```python
from build123d import *

# Parameters (mm, degrees)
SKETCH_1_W          = 196
SKETCH_1_H          = 221
EXTRUDE_1_DEPTH     = 3
EXTRUDE_2_DEPTH     = 128
FILLET_1_R          = 10
FILLET_2_R          = 10
SKETCH_3_R          = 3
SKETCH_3_R_2        = 40
CUT_EXTRUDE_1_DEPTH = 5
FILLET_3_R          = 10
FILLET_4_R          = 10
SKETCH_5_R          = 40
SKETCH_5_R_2        = 34
EXTRUDE_3_DEPTH     = 3
SKETCH_6_W          = 15
SKETCH_6_H          = 9
CUT_EXTRUDE_3_DEPTH = 159
EXTRUDE_4_DEPTH     = 10
EXTRUDE_4_2_DEPTH   = 10
EXTRUDE_4_3_DEPTH   = 10
EXTRUDE_4_4_DEPTH   = 10
EXTRUDE_6_DEPTH     = 1.5
FILLET_START        = -219
FILLET_6_DEPTH      = 216
FILLET_7_R          = 6.5
FILLET_8_R          = 8.5
FILLET_9_R          = 8.5
CUT_EXTRUDE_4_DEPTH = 10


with BuildPart() as part:
    # Sketch 1 → Extrude 1 (new body)
    with BuildSketch(Plane(origin=(0, 0, 0), x_dir=(1, 0, 0), z_dir=(0, 1, 0))):
        with Locations((98, 110.5)):
            Rectangle(SKETCH_1_W, SKETCH_1_H)
    extrude(amount=EXTRUDE_1_DEPTH)

    # Sketch 2 → Extrude 2 (add)
    with BuildSketch(Plane(origin=(0, 0, 0), x_dir=(1, 0, 0), z_dir=(0, 1, 0))):
        Polygon((3, 218), (3, 3), (20.5, 3), (20.5, 18), (24.5, 18), (24.5, 3), (24.5, 0), (0, 0), (0, 221), (196, 221), (196, 0), (171.5, 0), (171.5, 3), (171.5, 18), (175.5, 18), (175.5, 3), (193, 3), (193, 218), align=None)
    extrude(amount=-EXTRUDE_2_DEPTH)

    # Fillet 1
    fillet_1_edges = [part.edges().sort_by_distance(p)[0] for p in [
        (0, 3, -110.5),
    ]]
    fillet(fillet_1_edges, radius=FILLET_1_R)

    # Fillet 2
    fillet_2_edges = [part.edges().sort_by_distance(p)[0] for p in [
        (196, 3, -110.5),
    ]]
    fillet(fillet_2_edges, radius=FILLET_2_R)

    # Sketch 3 → Cut-Extrude 1 (cut)
    with BuildSketch(Plane(origin=(0, 0, -221), x_dir=(-1, 0, 0), z_dir=(0, 0, -1))):
        with Locations((-133.75, -9)):
            Circle(SKETCH_3_R)
        with Locations((-62.25, -9)):
            Circle(SKETCH_3_R)
        with Locations((-62.25, -80.5)):
            Circle(SKETCH_3_R)
        with Locations((-133.75, -80.5)):
            Circle(SKETCH_3_R)
        with Locations((-98, -44.75)):
            Circle(SKETCH_3_R_2)
    extrude(amount=-CUT_EXTRUDE_1_DEPTH, mode=Mode.SUBTRACT)

    # Fillet 3
    fillet_3_edges = [part.edges().sort_by_distance(p)[0] for p in [
        (193, 0, -110.5),
    ]]
    fillet(fillet_3_edges, radius=FILLET_3_R)

    # Fillet 4
    fillet_4_edges = [part.edges().sort_by_distance(p)[0] for p in [
        (3, 0, -110.5),
    ]]
    fillet(fillet_4_edges, radius=FILLET_4_R)

    # Sketch 5 → Extrude 3 (add)
    with BuildSketch(Plane(origin=(0, 0, -221), x_dir=(-1, 0, 0), z_dir=(0, 0, -1))):
        with Locations((-98, -44.75)):
            Circle(SKETCH_5_R)
        with Locations((-98, -44.75)):
            Circle(SKETCH_5_R_2, mode=Mode.SUBTRACT)
    extrude(amount=-EXTRUDE_3_DEPTH)

    # Sketch 6 → Cut-Extrude 3 (cut)
    with BuildSketch(Plane(origin=(175.5, 0, 0), x_dir=(0, 0, -1), z_dir=(1, 0, 0))):
        with Locations((10.5, -123.5)):
            Rectangle(SKETCH_6_W, SKETCH_6_H)
    extrude(amount=-CUT_EXTRUDE_3_DEPTH, mode=Mode.SUBTRACT)



with BuildPart() as body_2:
    # Sketch 10 → Extrude 4 (new body)
    with BuildSketch(Plane(origin=(0, -128, 0), x_dir=(-1, 0, 0), z_dir=(0, -1, 0))):
        Polygon((-5.5, 213.5), (-5.5, 143.5), (-9.5, 143.5), (-9.5, 209.5), (-35.5, 209.5), (-35.5, 213.5), align=None)
    extrude(amount=-EXTRUDE_4_DEPTH)


with BuildPart() as body_3:
    # Sketch 10 → Extrude 4 2 (new body)
    with BuildSketch(Plane(origin=(0, -128, 0), x_dir=(-1, 0, 0), z_dir=(0, -1, 0))):
        Polygon((-190.5, 213.5), (-160.5, 213.5), (-160.5, 209.5), (-186.5, 209.5), (-186.5, 143.5), (-190.5, 143.5), align=None)
    extrude(amount=-EXTRUDE_4_2_DEPTH)


with BuildPart() as body_4:
    # Sketch 10 → Extrude 4 3 (new body)
    with BuildSketch(Plane(origin=(0, -128, 0), x_dir=(-1, 0, 0), z_dir=(0, -1, 0))):
        Polygon((-16.5, 6.5), (-16.5, 10.5), (-9.5, 10.5), (-9.5, 116.5), (-5.5, 116.5), (-5.5, 6.5), align=None)
    extrude(amount=-EXTRUDE_4_3_DEPTH)


with BuildPart() as body_5:
    # Sketch 10 → Extrude 4 4 (new body)
    with BuildSketch(Plane(origin=(0, -128, 0), x_dir=(-1, 0, 0), z_dir=(0, -1, 0))):
        Polygon((-190.5, 6.5), (-179.5, 6.5), (-179.5, 10.5), (-186.5, 10.5), (-186.5, 116.5), (-190.5, 116.5), align=None)
    extrude(amount=-EXTRUDE_4_4_DEPTH)


with BuildPart() as part_1:
    add(part.part)

    add(body_2.part)  # Extrude 6 merges body 2

    add(body_3.part)  # Extrude 6 merges body 3

    add(body_4.part)  # Extrude 6 merges body 4

    add(body_5.part)  # Extrude 6 merges body 5
    # Sketch 11 → Extrude 6 (add)
    with BuildSketch(Plane(origin=(0, -118, 0), x_dir=(1, 0, 0), z_dir=(0, 1, 0))):
        Polygon((179.5, 6.5), (179.5, 3), (193, 3), (193, 218), (160.5, 218), (160.5, 209.5), (186.5, 209.5), (186.5, 10.5), (179.5, 10.5), align=None)
        Polygon((16.5, 10.5), (16.5, 3), (3, 3), (3, 218), (35.5, 218), (35.5, 209.5), (9.5, 209.5), (9.5, 10.5), align=None)
    extrude(amount=EXTRUDE_6_DEPTH)

    # Fillet 6: read off the stored shape, not the designer's step
    # Fillet 6 outline → Fillet 6 (add)
    with BuildSketch(Plane.XY.offset(FILLET_START)):
        with BuildLine():
            Line((3, -116.5), (9.5, -116.5))
            ThreePointArc((9.5, -116.5), (4.903805922, -114.596194078), (3, -110))
            Line((3, -110), (3, -116.5))
        make_face()
    extrude(amount=FILLET_6_DEPTH)

    # Fillet 7
    fillet_7_edges = [part_1.edges().sort_by_distance(p)[0] for p in [
        (193, -116.5, -110.5),
    ]]
    fillet(fillet_7_edges, radius=FILLET_7_R - 0.0001)  # a hair under: the kernel refuses the full size

    # Fillet 8
    # the kernel refuses this fillet: 8.5 mm, written as the material it adds along each edge
    with BuildSketch(Plane(origin=(-11.75, -116.5, -218), x_dir=(0, 1, 0), z_dir=(1, 0, 0))) as fillet_8_piece_1_section:
        with BuildLine():
            CenterArc((FILLET_8_R, FILLET_8_R), FILLET_8_R, 180, 90)
            Line((0, FILLET_8_R), (0, 0))
            Line((0, 0), (FILLET_8_R, 0))
        make_face()
    fillet_8_piece_1 = extrude(amount=47.25, mode=Mode.PRIVATE)
    fillet_8_piece_1 = split(fillet_8_piece_1, bisect_by=Plane(origin=(0, -116.5, -218), z_dir=(1, 0, 0)), keep=Keep.TOP, mode=Mode.PRIVATE)
    add(fillet_8_piece_1)

    # Fillet 9
    # the kernel refuses this fillet: 8.5 mm, written as the material it adds along each edge
    with BuildSketch(Plane(origin=(207.7501, -116.5, -218), x_dir=(0, 0, 1), z_dir=(-1, 0, 0))) as fillet_9_piece_1_section:
        with BuildLine():
            CenterArc((FILLET_9_R, FILLET_9_R), FILLET_9_R, 180, 90)
            Line((0, FILLET_9_R), (0, 0))
            Line((0, 0), (FILLET_9_R, 0))
        make_face()
    fillet_9_piece_1 = extrude(amount=47.2501, mode=Mode.PRIVATE)
    fillet_9_piece_1 = split(fillet_9_piece_1, bisect_by=Plane(origin=(196, -116.5, -218), z_dir=(-1, 0, 0)), keep=Keep.TOP, mode=Mode.PRIVATE)
    add(fillet_9_piece_1)

    # Sketch 12 → Cut-Extrude 4 (cut)
    with BuildSketch(Plane(origin=(0, -128, 0), x_dir=(-1, 0, 0), z_dir=(0, -1, 0))):
        Polygon((-16.5, 6.5), (-5.5, 6.5), (-5.5, 213.5), (-35.5, 213.5), (-35.5, 212.5), (-6.5, 212.5), (-6.5, 7.5), (-16.5, 7.5), align=None)
        Polygon((-190.5, 213.5), (-190.5, 6.5), (-179.5, 6.5), (-179.5, 7.5), (-189.5, 7.5), (-189.5, 212.5), (-160.5, 212.5), (-160.5, 213), (-160.5, 213.5), align=None)
    extrude(amount=-CUT_EXTRUDE_4_DEPTH, mode=Mode.SUBTRACT)


solid = part_1.part
```
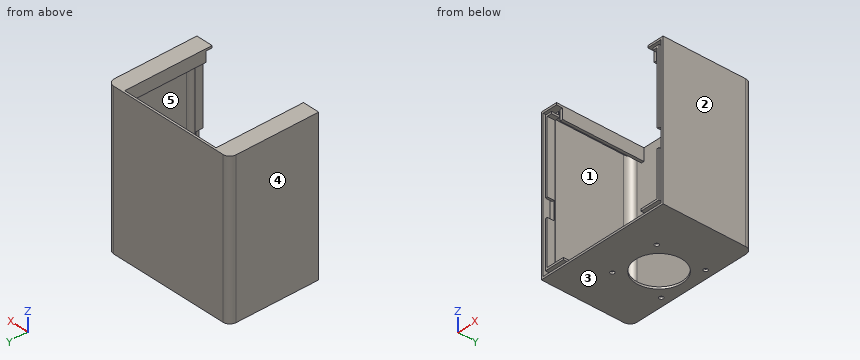
Design review of the part built by this model. Coordinates are the model's own, in mm. Face numbers are marked on the shaded views. A direction names the side the tool comes from. Give positions to 0.01 mm unless a question says otherwise; leave off trailing zeros. Write each loop counter-clockwise with the first axis right and the second up, starting at its lowest first coordinate (ties: lowest second). Pieces come first, ordered by that corner, then holes.
(1) Add section D-D (x = 74). Give the boundary of the cut face in (y, z).
Checked values:
outline: (-128, -221) - (-68.83, -221) - (-68.83, -218) - (-128, -218) - close; (-20.67, -221) - (3, -221) - (3, 0) - (0, 0) - (0, -218) - (-20.67, -218) - close
(2) Mouldability with a two-part tool opening along Z and no side actions: class the marked faces 3, 4 and 5 as +Z half, -Z half, draft (parallel to the pull), parting line (faces both ways), or undercut.
Checked values:
face 3: -Z half
face 4: draft
face 5: undercut
(3) Clearance check with flat-ended pins moving along their axes: pin 1 Ø5 at (x, z) = (37.5, -49.5) entering from -Y; pin 2 Ø12 at (x, y) = (161.5, -20) entering from +Z. State where each tip first meets the part, or that it passes through.
Checked values:
pin 1: stops at y = 0
pin 2: stops at z = -218
(4) Wall thickness on line 1 along X through (y, z) = (-80, -220); line 2 along Y through (x, z) = (62, -220); line 3 along Z through (x, y) = (11, -71.5): over which ranges is each line inside the solid? List them lowest first.
Checked values:
line 1: x = 0 to 59.29, 65.21 to 130.79, 136.71 to 196
line 2: y = -128 to -83.49, -77.51 to -11.99, -6.01 to 3
line 3: z = -221 to -218, -3 to 0
(5) Add section B-B (x = 122.5). Give the boundary of the cut face in (y, z), and give its area (3 significant figures).
Checked values:
outline: (-128, -221) - (-68.32, -221) - (-68.32, -218) - (-128, -218) - close; (-21.18, -221) - (3, -221) - (3, 0) - (0, 0) - (0, -218) - (-21.18, -218) - close
area: 906 mm2
(6) Tool access review of the marked faces 1 and 2: name each direction out of +Z, -Z, +X, -X, +Y, -Y from which nothing blocks a thin tool from reaching the whole face with its end or side.
Checked values:
face 1: none
face 2: +Z, -Z, +X, +Y, -Y
(7) Add section A-A (y = -54). Give the boundary of the cut face in (x, z), and give its area (3 significant figures).
Checked values:
outline: (0, -221) - (65.28, -221) - (65.28, -218) - (3, -218) - (3, -3) - (20.5, -3) - (20.5, -18) - (24.5, -18) - (24.5, 0) - (0, 0) - close; (130.72, -221) - (196, -221) - (196, 0) - (171.5, 0) - (171.5, -18) - (175.5, -18) - (175.5, -3) - (193, -3) - (193, -218) - (130.72, -218) - close
area: 1,950 mm2
